Design review of the part shown in the three views and the two pictorial views. Dimensions are in mm from the part's minimum x, y and z. Round coordinates to 2 decimals unless told otherwise and drop trailing zeros. Write each loop counter-clockwise with the first axis right and the second up, starting at its lowest first coordinate (ties: lowest second). Pieces come first, ordered by that corner, then holes. Notation, with made-up numbers: (-2, 66.5) - (16, 66.5) arc R9 cw to (16, 80.5) - close; hole circle Ø7 at (-33, 82.25). An arc over 180 degrees is marked (long way). One line per item, written item: value. Start each with the question number.
Q1. Add section D-D on z = 10.5. Write out the cut boundary in (x, y) (1 decimal).
Q2. Add section C-C on x = 76.5. Write out the cut boundary in (y, z) (1 decimal).
Q3. For probe 1 along X at (y, z) = (0.3, 4); probe 2 along Z at (x, y) = (46, 0.95); probe 3 along Z at (x, y) = (76.5, 0.65) (1 decimal), list the stretches that pass through material, from the lowest coordinate up.
Q4. Add section B-B on y = 0.6. Give the number of separate pieces and of enclosed holes in the cut face.
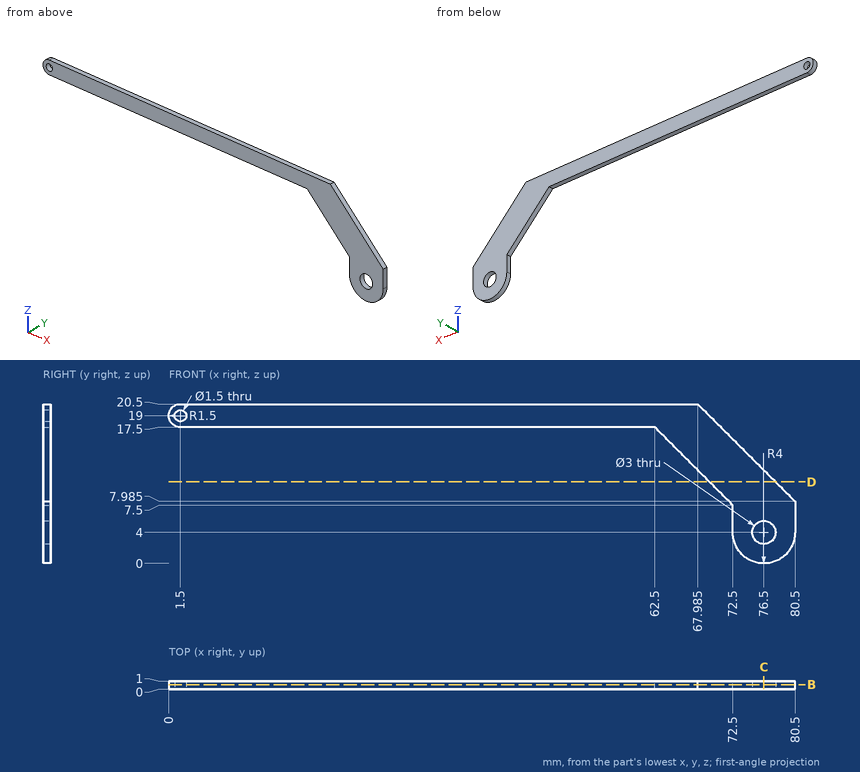
Result set:
1. outline: (69.5, 0) - (78, 0) - (78, 1) - (69.5, 1) - close
2. outline: (0, 0) - (1, 0) - (1, 2.5) - (0, 2.5) - close; (0, 5.5) - (1, 5.5) - (1, 12) - (0, 12) - close
3. probe 1: x = 72.5 to 75, 78 to 80.5
3. probe 2: z = 17.5 to 20.5
3. probe 3: z = 0 to 2.5, 5.5 to 12
4. separate pieces: 1
4. enclosed holes: 2
